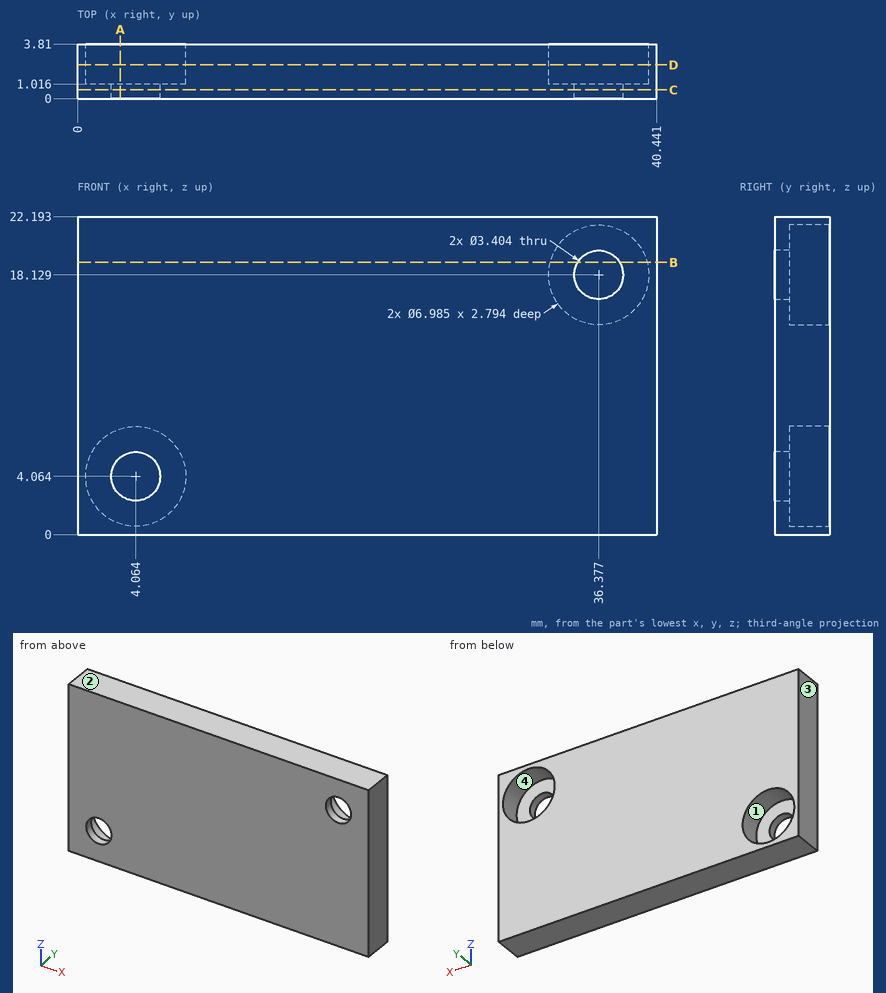
Geometry: see drawing. Coordinates: mm, zero at the bounding-box minimum. Round coordinates to 2 decimals unless told otherwise and drop trailing zeros. Loops run counter-clockwise (first coordinate to the right, second up) from the corner with the lowest first, then second, coordinate; pieces in that order, holes last. Notation, with made-up numbers: M 28.25,40.5 L 80.25,40.5 A20 cw 80.25,58.5 Z; hole C -4,58.25 d3. An arc over 180 degrees is marked long. Use a Markdown table: item, result. Add a question column.
1. Contact query for a flat-ended pin moving along its axis: pin 1 (2 mm diameter, centred on x = 4, z = 5, fed in from +Y). Output: stop coordinate, or through.
2. Cut plane C-C, the plane y = 0.6. Output: boundary loops of the cut face in (x, z) (1 decimal), and give its area (3 significant figures).
3. Cut plane A-A, the plane x = 3. Output: boundary loops of the cut face in (y, z).
4. Pull-direction query (X, two-part tool) for the marked faces 1, 2, 3 and 4; classes: +X half, -X half, draft (parallel to the pull), parting line (faces both ways), or undercut.
5. Ray query, line 1 along X through (y, z) = (0.75, 4) (1 decimal); line 2 along Z through (x, y) = (5, 2.1); line 3 along Z through (x, y) = (37, 2.2) (1 decimal). Return the intervals inside material, ascending. Write a range as [from, to].
6. Cut plane D-D, the plane y = 2.35. Output: boundary loops of the cut face in (x, z) (1 decimal).
7. Cut plane B-B, the plane z = 19. Output: boundary loops of the cut face in (x, y) (1 decimal), and give its area (3 significant figures).
Solution:
| question | item | result |
|---|---|---|
| 1 | pin 1 | stops at y = 1.02 |
| 2 | outline | M 0,0 L 40.4,0 L 40.4,22.2 L 0,22.2 Z; hole C 4.1,4.1 d3.4; hole C 36.4,18.1 d3.4 |
| 2 | area | 879 mm2 |
| 3 | outline | M 0,0 L 3.81,0 L 3.81,0.74 L 1.02,0.74 L 1.02,2.74 L 0,2.74 Z; M 0,5.39 L 1.02,5.39 L 1.02,7.39 L 3.81,7.39 L 3.81,22.19 L 0,22.19 Z |
| 4 | face 1 | undercut |
| 4 | face 2 | draft |
| 4 | face 3 | -X half |
| 4 | face 4 | undercut |
| 5 | line 1 | x = [0, 2.4], [5.8, 40.4] |
| 5 | line 2 | z = [0, 0.7], [7.43, 22.19] |
| 5 | line 3 | z = [0, 14.7], [21.6, 22.2] |
| 6 | outline | M 0,0 L 40.4,0 L 40.4,22.2 L 0,22.2 Z; hole C 4.1,4.1 d7; hole C 36.4,18.1 d7 |
| 7 | outline | M 0,0 L 34.9,0 L 34.9,1 L 33,1 L 33,3.8 L 0,3.8 Z; M 37.8,0 L 40.4,0 L 40.4,3.8 L 39.8,3.8 L 39.8,1 L 37.8,1 Z |
| 7 | area | 132 mm2 |
